```python
from build123d import *

# Parameters (mm, degrees)
SKETCH1_R                                           = 25
SKETCH1_R_2                                         = 19
BOSS_EXTRUDE1_DEPTH                                 = 5
SKETCH2_R                                           = 25
BOSS_EXTRUDE2_DEPTH                                 = 10
FILLET1_R                                           = 5
CBORE_FOR_3_BINDING_HEAD_MACHINE_SCREW1_D           = 3.048
CBORE_FOR_3_BINDING_HEAD_MACHINE_SCREW1_CBORE_D     = 5.95376
CBORE_FOR_3_BINDING_HEAD_MACHINE_SCREW1_CBORE_DEPTH = 1.4986
CUT_EXTRUDE1_START                                  = -3
CUT_EXTRUDE1_DEPTH                                  = 10
SCALE1_SCALE                                        = 1.5


with BuildPart() as part:
    # Sketch1 → Boss-Extrude1 (new body)
    with BuildSketch(Plane.XY):
        Circle(SKETCH1_R)
        Circle(SKETCH1_R_2, mode=Mode.SUBTRACT)
    extrude(amount=BOSS_EXTRUDE1_DEPTH)

    # Sketch2 → Boss-Extrude2 (add)
    with BuildSketch(Plane.XY.offset(5)):
        Circle(SKETCH2_R)
    extrude(amount=BOSS_EXTRUDE2_DEPTH)

    # Fillet1
    fillet1_edges = [part.edges().sort_by_distance(p)[0] for p in [
        (-25, 0, 15),
        (-19, 0, 5),
    ]]
    fillet(fillet1_edges, radius=FILLET1_R - 0.0001)  # a hair under: the kernel refuses the full size

    # CBORE for #3 Binding Head Machine Screw1 (through all)
    with Locations(Plane.XY.offset(15)):
        with Locations((0, 22.435050854), (0, -22.295918756), (22.400267829, 0), (-22.608965977, 0)):
            CounterBoreHole(CBORE_FOR_3_BINDING_HEAD_MACHINE_SCREW1_D / 2, CBORE_FOR_3_BINDING_HEAD_MACHINE_SCREW1_CBORE_D / 2, CBORE_FOR_3_BINDING_HEAD_MACHINE_SCREW1_CBORE_DEPTH)

    # Sketch15 → Cut-Extrude1 (cut)
    with BuildSketch(Plane(origin=(0, 0, 5), x_dir=(-1, 0, 0), z_dir=(0, 0, -1)).offset(CUT_EXTRUDE1_START)):
        with BuildLine():
            Line((1.676226843, 1.500920907), (2.037127027, 4.807341739))
            Line((2.037127027, 4.807341739), (-0.948609283, 5.133238785))
            Line((-0.948609283, 5.133238785), (-1.309172026, 1.829909453))
            ThreePointArc((-1.309172026, 1.829909453), (-1.94216249, 1.136003901), (-2.236715327, 0.244140421))
            ThreePointArc((-2.236715327, 0.244140421), (-2.141502308, -0.690266516), (-1.673115077, -1.504388892))
            Line((-1.673115077, -1.504388892), (-2.03367782, -4.807718225))
            Line((-2.03367782, -4.807718225), (0.952058491, -5.133615271))
            Line((0.952058491, -5.133615271), (1.312958675, -1.827194439))
            ThreePointArc((1.312958675, -1.827194439), (1.943337692, -1.133992334), (2.236715327, -0.244140421))
            ThreePointArc((2.236715327, -0.244140421), (2.142215878, 0.688048787), (1.676226843, 1.500920907))
        make_face()
    extrude(amount=-CUT_EXTRUDE1_DEPTH, mode=Mode.SUBTRACT)


with BuildPart() as part_1:
    # Scale1: scaled about (-0.000833746, 0.000507816, 8.367914089)
    add(part.part.scale(SCALE1_SCALE).moved(Location((0.000416873, -0.000253908, -4.183957044))))


solid = part_1.part
```
Part model, mm, in its own coordinate system. A direction names the side the tool comes from. Round coordinates to 2 decimals unless told otherwise and drop trailing zeros. Write each loop counter-clockwise with the first axis right and the second up, starting at its lowest first coordinate (ties: lowest second). Pieces come first, ordered by that corner, then holes. Notation, with made-up numbers: M 63.25,68 L 83.25,68 A25 cw 83.25,87 Z; hole C 52.5,26.25 d5. An arc over 180 degrees is marked long. One line per question, with ' | ' between items.
(1) 3-axis set-ups, long thin cutter, end or side, ignore diameter. For faces 1 (the face through (0.3, 35.92, 5.8)), 2 (the face through (2.777, -4.7, 12.993)): which of +Z, -Z, +X, -X, +Y, -Y reach the whole face in a straight line?
Answer key:
face 1: +Z, -Z | face 2: +Z
(2) Saw through at B-B on z = 6.25. Write the cut outline in (x, y), then the cut area to 3 significant figures.
Answer key:
outline: C 0,0 d75; hole C -33.91,0 d4.57; hole C 0,-33.44 d4.57; hole C 0,33.65 d4.57; hole C 33.6,0 d4.57 | area: 4,350 mm^2
(3) Pin check, flat tips, straight feed: pin 1 (4.5 mm diameter, centred on x = -32.5, y = -1, fed in from +Z); pin 2 (10 mm diameter, centred on x = 23.5, z = 1, fed in from +Y); pin 3 (2 mm diameter, centred on x = 0, y = -2, fed in from +Z). Stop position of each tip, or through.
Answer key:
pin 1: stops at z = 16.07 | pin 2: stops at y = 32.62 | pin 3: stops at z = 7.82
(4) Probe line 1 along Y through (x, z) = (1, 5.25); line 2 along X through (y, z) = (0.5, -2); line 3 along X through (y, z) = (-2, 10.25). List the from-to ranges inside material, lowest first.
Answer key:
line 1: y = -37.49 to -35.5, -31.39 to 31.6, 35.71 to 37.49 | line 2: x = -37.5 to -36.14, -31.68 to -28.17, 28.17 to 31.37, 35.83 to 37.5 | line 3: x = -37.45 to -35.02, -32.81 to -2.72, 2.72 to 32.49, 34.71 to 37.45
(5) Saw through at C-C on z = 0.5. Write the cut outline in (x, y).
Answer key:
outline: C 0,0 d75; hole C -33.91,0 d4.57; hole C 0,0 d53.72; hole C 0,-33.44 d4.57; hole C 0,33.65 d4.57; hole C 33.6,0 d4.57
(6) Saw through at A-A on z = 13.25. Write the cut outline in (x, y) (3 decimals), then the cut area to 3 significant figures.
Answer key:
outline: C 0,0 d74.188; hole C -33.913,0 d4.572; hole M -3.055,7.211 L -2.514,2.251 A3.375 ccw -1.969,-2.741 L -1.428,-7.701 L 3.051,-7.212 L 2.51,-2.257 A3.375 ccw 1.964,2.745 L 1.423,7.7 Z; hole C 0,-33.444 d4.572; hole C 0,33.652 d4.572; hole C 33.601,0 d4.572 | area: 4,180 mm^2
